Geometry: final body of the model. Coordinates: model frame, mm. Round coordinates to 2 decimals unless told otherwise and drop trailing zeros. Write each loop counter-clockwise with the first axis right and the second up, starting at its lowest first coordinate (ties: lowest second). Pieces come first, ordered by that corner, then holes. Notation, with made-up numbers: (-8.75, -27.5) - (37.25, -27.5) arc R29 cw to (37.25, 10.5) - close; hole circle Ø4 at (21, 18). An arc over 180 degrees is marked (long way). Use a Markdown table: item, result. Add a question column.
```python
from build123d import *

# Parameters (mm, degrees)
F0_R     = 50
F1_DEPTH = 50
F2_DEPTH = 50
F3_SIZE  = 2
F4_T     = -1
F5_R     = 0.49999


# Not quite as in the source:
# - a fillet or chamfer is up to 0.001 mm smaller than in the source, because OpenCascade refuses the exact size


with BuildPart() as f1:
    # F0 (on Top) → F1 (new body)
    with BuildSketch(Plane.XY):
        Circle(F0_R)
    extrude(amount=F1_DEPTH)

    # F2 (add): a face of the model
    f2_faces = [f1.faces().sort_by_distance(p)[0] for p in [
        (0, 0, 0),
    ]]
    extrude(f2_faces, amount=F2_DEPTH)

    # F3
    f3_edges = [f1.edges().sort_by_distance(p)[0] for p in [
        (-50, 0, -50),
    ]]
    chamfer(f3_edges, length=F3_SIZE)

    # F4
    f4_openings = [f1.faces().sort_by_distance(p)[0] for p in [
        (0, 0, 50),
    ]]
    offset(amount=F4_T, openings=f4_openings)

    # F5 (radius 0.5 in the source; OpenCascade refuses exactly that, so slightly less here)
    f5_edges = [f1.edges().sort_by_distance(p)[0] for p in [
        (-50, 0, 50),
        (-49, 0, 50),
    ]]
    fillet(f5_edges, radius=F5_R)


solid = f1.part
```
1) Pin query (flat end, axial travel): P1, Ø6, axis at x = -16, z = -37.5, coming from the -Y side; P2, Ø1, axis at y = 33, z = -16.5, coming from the -X side; P3, Ø4, axis at x = -23, z = -2, coming from the -Y side. Return the tip coordinate at first contact, or that it passes through.
2) Material intervals for L1, parallel to Y at x = 0, z = 19; L2, parallel to Z at x = 8.5, y = 15; L3, parallel to Y at x = 40.5, z = -13, sorted ascending. Write a range as from..to.
3) Section C-C, the plane z = -14. Return the cut outline in (x, y).
4) Draft query along X for faces 1 (the flat face through (-1, 1, -49)), 2 (the flat face through (-1, 1, -50)), 3 (the cylindrical face through (47.69, 15.02, 1.43)). Return one class per face: released by +X, released by -X, zero draft, split by the parting line, or undercut.
Output values:
| question | item | result |
|---|---|---|
| 1 | P1 | stops at y = -48.28 |
| 1 | P2 | stops at x = -38 |
| 1 | P3 | stops at y = -45.38 |
| 2 | L1 | y = -50..-49, 49..50 |
| 2 | L2 | z = -50..-49 |
| 2 | L3 | y = -29.32..-27.58, 27.58..29.32 |
| 3 | outline | circle Ø100 at (0, 0); hole circle Ø98 at (0, 0) |
| 4 | face 1 | undercut |
| 4 | face 2 | zero draft |
| 4 | face 3 | split by the parting line |
